from build123d import *

# Parameters (mm, degrees)
SKETCH1_R               = 27.5
SKETCH1_R_2             = 23.8
BOSS_EXTRUDE1_DEPTH     = 3
CUT_EXTRUDE1_REACH      = 63.565
CUT_EXTRUDE1_END_RADIUS = 23.8


with BuildPart() as part:
    # Sketch1 → Boss-Extrude1 (new body)
    with BuildSketch(Plane(origin=(0, 0, 0), x_dir=(1, 0, 0), z_dir=(0, 1, 0))):
        with Locations(Location((0, 0, 0), (0, 0, 270))):
            Circle(SKETCH1_R)
        with Locations(Location((0, 0, 0), (0, 0, 270))):
            Circle(SKETCH1_R_2, mode=Mode.SUBTRACT)
    extrude(amount=BOSS_EXTRUDE1_DEPTH)

    # Cut-Extrude1: up to this cylinder (the profile starts outside it)
    cut_extrude1_end = Plane(origin=(0, 1.5, 0), z_dir=(0, -1, 0)) * Cylinder(CUT_EXTRUDE1_END_RADIUS, 175.73, mode=Mode.PRIVATE)
    # Sketch2 → Cut-Extrude1 (cut, up to the surface)
    with BuildSketch(Plane.XY.offset(27.5), mode=Mode.PRIVATE) as cut_extrude1_sk1:
        Polygon((-2.627763182, 0), (2.56838924, 3), (4.06838924, 3), (-1.127763182, 0), align=None)
    cut_extrude1_tool1 = extrude(cut_extrude1_sk1.sketch, amount=-CUT_EXTRUDE1_REACH, mode=Mode.PRIVATE) - cut_extrude1_end
    add(cut_extrude1_tool1.solids().sort_by_distance((0.720313, 1.5, 27.5))[0], mode=Mode.SUBTRACT)


solid = part.part
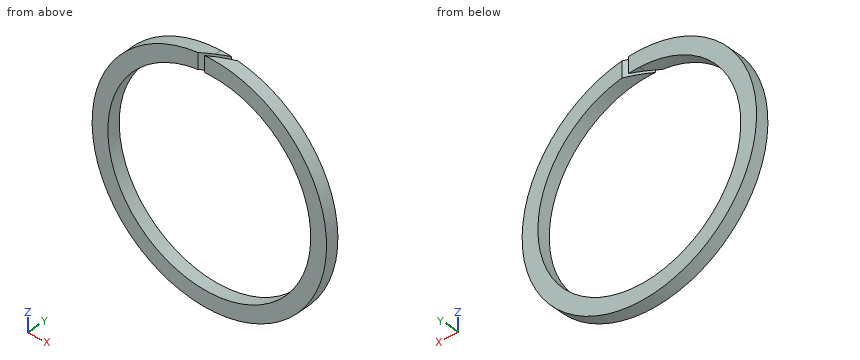
Geometry: final body of the model. Coordinates: model frame, mm. Give positions to 0.01 mm unless a question says otherwise; leave off trailing zeros. Write each loop counter-clockwise with the first axis right and the second up, starting at its lowest first coordinate (ties: lowest second). Pieces come first, ordered by that corner, then holes. Notation, with made-up numbers: (62, -36.75) -> (92, -36.75) arc R36 ccw to (92, -2.75) -> close; hole circle Ø11 at (11, -32.5). An arc over 180 degrees is marked (long way). Answer in a Markdown table with one row per item.
(1) Ray query, line 1 along X through (y, z) = (2.45, 0); line 2 along X through (y, z) = (1.55, -20.5). Return the intervals inside material, ascending. Write a range as [from, to].
Answers below:
| item | result |
|---|---|
| line 1 | [-27.5, -23.8], [23.8, 27.5] |
| line 2 | [-18.33, -12.09], [12.09, 18.33] |
(2) Section query C-C on y = 2.45. Return loops of the section in (x, z).
Answers below:
| item | result |
|---|---|
| outline | (1.62, 23.75) -> (1.62, 27.45) arc R27.5 ccw (long way) to (3.12, 27.32) -> (3.12, 23.6) arc R23.8 cw (long way) to start |
(3) Pin query (flat end, axial travel): pin 1 (5 mm diameter, centred on x = 5.5, z = -19, fed in from +Y); pin 2 (1 mm diameter, centred on x = -13, z = -19.5, fed in from -Y). Return the tip coordinate at first contact, or that it passes through.
Answers below:
| item | result |
|---|---|
| pin 1 | through |
| pin 2 | y = 0 |
(4) Section query B-B on x = 21. Return loops of the section in (y, z), then the cut area to 3 significant figures.
Answers below:
| item | result |
|---|---|
| outline | (0, -17.76) -> (3, -17.76) -> (3, -11.2) -> (0, -11.2) -> close; (0, 11.2) -> (3, 11.2) -> (3, 17.76) -> (0, 17.76) -> close |
| area | 39.3 mm^2 |
(5) Section query A-A on z = 0. Return loops of the section in (x, y).
Answers below:
| item | result |
|---|---|
| outline | (-27.5, 0) -> (-23.8, 0) -> (-23.8, 3) -> (-27.5, 3) -> close; (23.8, 0) -> (27.5, 0) -> (27.5, 3) -> (23.8, 3) -> close |
